Drawing for the job (mm, zero at the part's lowest x, y, z). A direction names the side the tool comes from. Round coordinates to 2 decimals unless told otherwise and drop trailing zeros. Order: outer loops, then holes, each group sorted by start corner. A loop starts at its lowest first (then second) coordinate and runs counter-clockwise, first axis right, second up. Notation, with made-up numbers: M 51.5,-17 L 81.5,-17 A10 ccw 81.5,-6 Z; hole C -12.75,15.5 d10. An arc over 180 degrees is marked long. One line per item, written item: value. Start each with the question number.
Item 1: Probe L1, parallel to X at y = 18.5, z = 7.25; L2, parallel to X at y = 15.25, z = 11.5; L3, parallel to X at y = 16, z = 6.75. List the from-to ranges inside material, lowest first.
Item 2: Pin check, flat tips, straight feed: pin 1 (10 mm diameter, centred on x = 25.5, z = 13.5, fed in from +Y); pin 2 (1.5 mm diameter, centred on y = 17.5, z = 4, fed in from -X); pin 3 (3 mm diameter, centred on x = 5.5, y = 9, fed in from -Z). Stop position of each tip, or through.
Item 3: Two-plate mould, pull along X, no slides. Class the marked faces 4, 5 and 6: +X half, -X half, draft (parallel to the pull), parting line (faces both ways), or undercut.
Item 4: Band-saw the part on D-D, the plane x = 36. Write the cut outline in (y, z), then the cut area to 3 significant figures.
Item 5: Band-saw the part on C-C, the plane x = 19. Write the cut outline in (y, z), then the cut area to 3 significant figures.
Item 6: Band-saw the part on A-A, the plane z = 10. Write the cut outline in (x, y).
Item 7: Tool access for the marked faces 1, 2 and 3: list every direction of +Z, -Z, +X, -X, +Y, -Y with a clear straight run to the whole face (end or side of a thin tool).
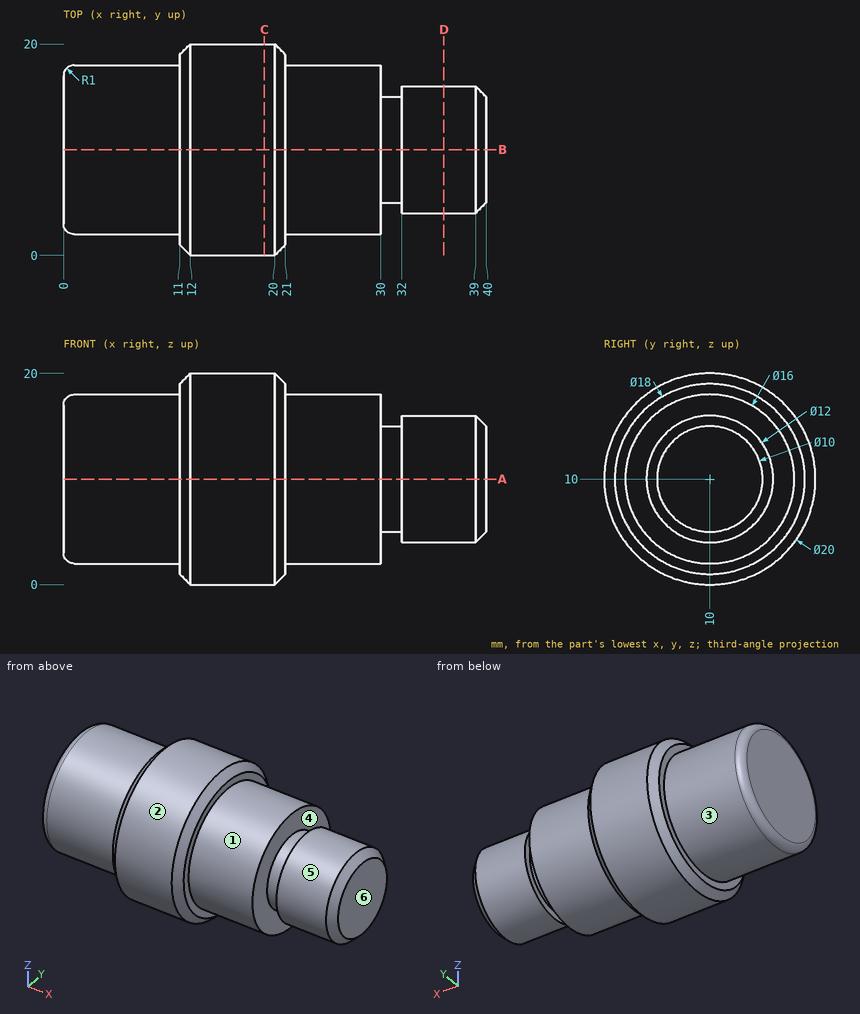
Output:
1. L1: x = 11 to 21
1. L2: x = 0 to 30, 32 to 39.54
1. L3: x = 0 to 30
2. pin 1: stops at y = 19.07
2. pin 2: stops at x = 11
2. pin 3: stops at z = 2
3. face 4: undercut
3. face 5: draft
3. face 6: +X half
4. outline: C 10,10 d12
4. area: 113 mm²
5. outline: C 10,10 d20
5. area: 314 mm²
6. outline: M 0,3 A1 ccw 1,2 L 11,2 L 11,1 L 12,0 L 20,0 L 21,1 L 21,2 L 30,2 L 30,5 L 32,5 L 32,4 L 39,4 L 40,5 L 40,15 L 39,16 L 32,16 L 32,15 L 30,15 L 30,18 L 21,18 L 21,19 L 20,20 L 12,20 L 11,19 L 11,18 L 1,18 A1 ccw 0,17 Z
7. face 1: +X
7. face 2: +X, -X
7. face 3: -X
